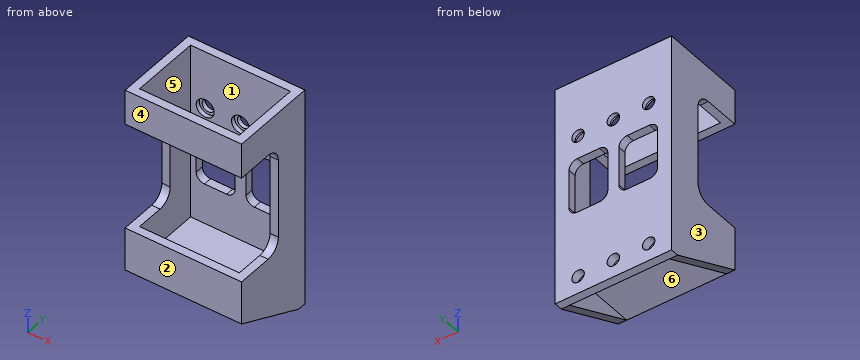
```python
from build123d import *

# Parameters (mm, degrees)
F0_W      = 36
F0_H      = 12.73
F0_W_2    = 3
F1_DEPTH  = 31
F0_H_2    = 38.81
F2_DEPTH  = 13
F0_R      = 2.25
F3_DEPTH  = 3
F4_DEPTH  = 3
F5_DEPTH  = 31
F7_DEPTH  = 12.73
F8_W      = 36
F8_H      = 25
F9_DEPTH  = 25
F11_DEPTH = 25
F13_DEPTH = 25
F14_R     = 3.25
F14_R_2   = 2.25
F15_DEPTH = 1.5
F16_W     = 14
F16_H     = 20.04
F17_DEPTH = 25
F18_R     = 3
F19_R     = 5


# Not quite as in the source:
# - a feature names something its author has since deleted; it is built from what else it names


with BuildPart() as f1:
    # F0 (on Front) → F1 (new body)
    with BuildSketch(Plane.XZ):
        with Locations((21, 73.635)):
            Rectangle(F0_W, F0_H)
        with Locations((1.5, 73.635)):
            Rectangle(F0_W_2, F0_H)
        with Locations((40.5, 73.635)):
            Rectangle(F0_W_2, F0_H)
    extrude(amount=F1_DEPTH)



with BuildPart() as f1b:
    # F0 (on Front) → F1, piece 2 (new body)
    with BuildSketch(Plane.XZ):
        with Locations((40.5, 22.095)):
            Rectangle(F0_W_2, F0_H)
        with Locations((21, 22.095)):
            Rectangle(F0_W, F0_H)
        with Locations((1.5, 22.095)):
            Rectangle(F0_W_2, F0_H)
        Polygon((0, 15.73), (0, 12.73), (3, 12.73), (39, 12.73), (42, 12.73), (42, 15.73), (39, 15.73), (3, 15.73), align=None)
    extrude(amount=F1_DEPTH)


with BuildPart() as f1_1:
    add(f1.part)

    add(f1b.part)  # F2 merges F1b
    # F0 (on Front) → F2 (join)
    with BuildSketch(Plane.XZ):
        with Locations((40.5, 47.865)):
            Rectangle(F0_W_2, F0_H_2)
        with Locations((1.5, 47.865)):
            Rectangle(F0_W_2, F0_H_2)
    extrude(amount=F2_DEPTH)

    # F0 (on Front) → F3 (join)
    with BuildSketch(Plane.XZ):
        with Locations((21, 6.365)):
            Rectangle(F0_W, F0_H)
        with Locations((8.27, 6.37)):
            Circle(F0_R, mode=Mode.SUBTRACT)
        with Locations((21, 6.37)):
            Circle(F0_R, mode=Mode.SUBTRACT)
        with Locations((33.73, 6.37)):
            Circle(F0_R, mode=Mode.SUBTRACT)
    extrude(amount=F3_DEPTH)

    # F0 (on Front) → F4 (join)
    with BuildSketch(Plane.XZ):
        with Locations((21, 47.865)):
            Rectangle(F0_W, F0_H_2)
        with Locations((8.27, 58.87)):
            Circle(F0_R, mode=Mode.SUBTRACT)
        with Locations((21, 58.87)):
            Circle(F0_R, mode=Mode.SUBTRACT)
        with Locations((33.73, 58.87)):
            Circle(F0_R, mode=Mode.SUBTRACT)
    extrude(amount=F4_DEPTH)

    # F0 (on Front) → F5 (join)
    with BuildSketch(Plane.XZ):
        with Locations((40.5, 6.365)):
            Rectangle(F0_W_2, F0_H)
        with Locations((1.5, 6.365)):
            Rectangle(F0_W_2, F0_H)
    extrude(amount=F5_DEPTH)

    # F6 (on face) → F7 (cut)
    with BuildSketch(Plane.XY.offset(28.46)):
        Polygon((39, -3), (3, -3), (3, -13), (3, -28), (39, -28), (39, -13), align=None)
    extrude(amount=-F7_DEPTH, mode=Mode.SUBTRACT)

    # F8 (on face) → F9 (cut)
    with BuildSketch(Plane.XY.offset(80)):
        with Locations((21, -15.5)):
            Rectangle(F8_W, F8_H)
    extrude(amount=-F9_DEPTH, mode=Mode.SUBTRACT)

    # F10 (on face) → F11 (cut)
    with BuildSketch(Plane.YZ.offset(3)):
        Polygon((-3, 0), (-31, 12.73), (-31, 0), align=None)
    extrude(amount=-F11_DEPTH, mode=Mode.SUBTRACT)

    # F12 (on face) → F13 (cut)
    with BuildSketch(Plane(origin=(39, 0, 0), x_dir=(0, -1, 0), z_dir=(-1, 0, 0))):
        Polygon((31, 0), (31, 12.73), (3, 0), align=None)
    extrude(amount=-F13_DEPTH, mode=Mode.SUBTRACT)

    # F14 (on face) → F15 (cut)
    with BuildSketch(Plane.XZ.offset(3)):
        with Locations((8.27, 58.87)):
            Circle(F14_R)
        with Locations((8.27, 58.87)):
            Circle(F14_R_2, mode=Mode.SUBTRACT)
        with Locations((21, 58.87)):
            Circle(F14_R)
        with Locations((21, 58.87)):
            Circle(F14_R_2, mode=Mode.SUBTRACT)
        with Locations((33.73, 58.87)):
            Circle(F14_R)
        with Locations((33.73, 58.87)):
            Circle(F14_R_2, mode=Mode.SUBTRACT)
    extrude(amount=-F15_DEPTH, mode=Mode.SUBTRACT)

    # F16 (on face) → F17 (cut)
    with BuildSketch(Plane.XZ.offset(3)):
        with Locations((12, 40.48)):
            Rectangle(F16_W, F16_H)
        with Locations((30, 40.48)):
            Rectangle(F16_W, F16_H)
    extrude(amount=-F17_DEPTH, mode=Mode.SUBTRACT)

    # F18
    f18_edges = [f1_1.edges().sort_by_distance(p)[0] for p in [
        (5, -1.5, 50.5),
        (5, -1.5, 30.46),
        (37, -1.5, 30.46),
        (23, -1.5, 30.46),
        (19, -1.5, 30.46),
        (19, -1.5, 50.5),
        (23, -1.5, 50.5),
        (37, -1.5, 50.5),
    ]]
    fillet(f18_edges, radius=F18_R)

    # F19
    f19_edges = [f1_1.edges().sort_by_distance(p)[0] for p in [
        (1.5, -13, 67.27),
        (40.5, -13, 67.27),
        (1.5, -13, 28.46),
        (40.5, -13, 28.46),
    ]]
    fillet(f19_edges, radius=F19_R)


solid = f1_1.part
```
Input: part model. Units: mm. Frame: model coordinates. Face numbers are marked on the shaded views. A direction names the side the tool comes from. Coordinates: 2 decimals unless noted, no trailing zeros. Write each loop counter-clockwise with the first axis right and the second up, starting at its lowest first coordinate (ties: lowest second). Pieces come first, ordered by that corner, then holes. Notation, with made-up numbers: (-30.5, -40) -> (-14.5, -40) arc R12 cw to (-14.5, -23) -> close; hole circle Ø4 at (15, 23.25). An arc over 180 degrees is marked (long way). Answer as a JSON object with one key per item and string values.
1. Section C-C on x = 13. Return the cut outline in (y, z), then the cut area to 3 significant figures.
Result set:
{"outline": "(-31, 12.73) -> (-3, 12.73) -> (-3, 0) -> (0, 0) -> (0, 30.46) -> (-3, 30.46) -> (-3, 15.73) -> (-28, 15.73) -> (-28, 28.46) -> (-31, 28.46) -> close; (-31, 67.27) -> (-28, 67.27) -> (-28, 80) -> (-31, 80) -> close; (-3, 50.5) -> (0, 50.5) -> (0, 80) -> (-3, 80) -> close", "area": "340 mm2"}
2. Access query for the marked faces 4, 5 and 6. Directions: +Z, -Z, +X, -X, +Y, -Y. A direction counts if a zero-diameter tool reaches every point of the face in a straight line with its end or side. Return the directions, or none.
Result set:
{"face 4": "+Z, -Z, +X, -X, -Y", "face 5": "+Z", "face 6": "-Z, -Y"}
3. Section D-D on y = -14.5. Return the cut outline in (x, z), then the cut area to 3 significant figures.
Result set:
{"outline": "(0, 5.23) -> (3, 5.23) -> (3, 12.73) -> (39, 12.73) -> (39, 5.23) -> (42, 5.23) -> (42, 29.89) -> (39, 29.89) -> (39, 15.73) -> (3, 15.73) -> (3, 29.89) -> (0, 29.89) -> close; (0, 65.84) -> (3, 65.84) -> (3, 80) -> (0, 80) -> close; (39, 65.84) -> (42, 65.84) -> (42, 80) -> (39, 80) -> close", "area": "341 mm2"}
4. First-contact query: P1, Ø11, axis at x = 22, z = 34.5, coming from the -Y side; P2, Ø10, axis at x = 24, z = 43, coming from the +Y side; P3, Ø3, axis at x = 36.5, y = -6, coming from the +Z side; P4, Ø2.5, axis at x = 1, z = 52.5, coming from the -Y side. Flat tips, straight axial feed; report the tip coordinate or a pass-through.
Result set:
{"P1": "stops at y = -3", "P2": "stops at y = 0", "P3": "stops at z = 15.73", "P4": "stops at y = -13"}
5. Section A-A on x = 21. Return the cut outline in (y, z), then the cut area to 3 significant figures.
Result set:
{"outline": "(-31, 12.73) -> (-3, 12.73) -> (-3, 8.62) -> (0, 8.62) -> (0, 56.62) -> (-1.5, 56.62) -> (-1.5, 55.62) -> (-3, 55.62) -> (-3, 15.73) -> (-28, 15.73) -> (-28, 28.46) -> (-31, 28.46) -> close; (-31, 67.27) -> (-28, 67.27) -> (-28, 80) -> (-31, 80) -> close; (-3, 0) -> (0, 0) -> (0, 4.12) -> (-3, 4.12) -> close; (-3, 62.12) -> (-1.5, 62.12) -> (-1.5, 61.12) -> (0, 61.12) -> (0, 80) -> (-3, 80) -> close", "area": "370 mm2"}
6. Material intervals for line 1 (Z direction, x = 8, y = -2); line 2 (Z direction, x = 21, y = -0.65); line 3 (X direction, y = -22, z = 69.5), sorted ascending. Write a range as from..to.
Result set:
{"line 1": "z = 0..4.14, 8.6..30.46, 50.5..55.63, 62.11..80", "line 2": "z = 0..4.12, 8.62..56.62, 61.12..80", "line 3": "x = 0..3, 39..42"}
7. Mould query, pull axis X, two halves, no side actions, for the marked faces 1, 2 and 3. Classes: released by +X, released by -X, zero draft, split by the parting line, or undercut.
Result set:
{"face 1": "undercut", "face 2": "zero draft", "face 3": "released by -X"}
8. Section B-B on z = 58.87. Count the separate pieces of the cut face and the enclosed holes in it, then the cut area to 4 significant figures.
Result set:
{"separate pieces": "4", "enclosed holes": "0", "area": "136.5 mm2"}
